```python
from build123d import *

# Parameters (mm, degrees)
SKETCH_1_W          = 35
SKETCH_1_H          = 10
SKETCH_1_R          = 2.1
EXTRUDE_1_DEPTH     = 2.5
EXTRUDE_2_DEPTH     = 2.5
SKETCH_2_3_R        = 1.6
CUT_EXTRUDE_1_DEPTH = 73.650942584
CHAMFER_1_SIZE      = 24.494897428
CHAMFER_1_SIZE_2    = 30
FILLET_1_R          = 2


with BuildPart() as part:
    # 草图1 → 凸台-拉伸1 (new body)
    with BuildSketch(Plane(origin=(0, 0, 0), x_dir=(1, 0, 0), z_dir=(0, 1, 0))):
        Rectangle(SKETCH_1_W, SKETCH_1_H)
        with Locations(Location((-7.5, 0, 0), (0, 0, 270))):
            Circle(SKETCH_1_R, mode=Mode.SUBTRACT)
        with Locations(Location((7.5, 0, 0), (0, 0, 270))):
            Circle(SKETCH_1_R, mode=Mode.SUBTRACT)
    extrude(amount=EXTRUDE_1_DEPTH)

    # 草图2 → 凸台-拉伸2 (add)
    with BuildSketch(Plane(origin=(0, 2.5, 0), x_dir=(1, 0, 0), z_dir=(0, 1, 0))):
        Polygon((-63.004240202, 2.548597579), (-52.651478398, -36.088435473), (17.5, -17.291403488), (17.5, -5), (-17.5, -5), (-17.5, 14.741421993), align=None)
    extrude(amount=-EXTRUDE_2_DEPTH)

    # 草图2<3> → 切除-拉伸1 (cut, through all)
    with BuildSketch(Plane(origin=(0, 2.5, 0), x_dir=(1, 0, 0), z_dir=(0, 1, 0))):
        with Locations(Location((-30.144179737, -4.175718463, 0), (0, 0, 270))):
            Circle(SKETCH_2_3_R)
        with Locations(Location((-24.967798835, -23.494234988, 0), (0, 0, 270))):
            Circle(SKETCH_2_3_R)
    extrude(amount=-CUT_EXTRUDE_1_DEPTH, mode=Mode.SUBTRACT)

    # 倒角1
    # the kernel refuses this chamfer: 30, 24.494897428 mm, written as the material it takes off along each edge
    with BuildSketch(Plane(origin=(-17.5, 79.650489639, -14.741421993), x_dir=(0.04137655931612181, 0, 0.999143623479207), z_dir=(0, -1, 0))) as chamfer_1_piece_1_section:
        Polygon((CHAMFER_1_SIZE * 0.999143623472, CHAMFER_1_SIZE * 0.0413765593158), (CHAMFER_1_SIZE_2 * 0.218630711303, CHAMFER_1_SIZE_2 * 0.975807671662), (0, 0), align=None)
    chamfer_1_piece_1 = extrude(amount=156.800979278, mode=Mode.PRIVATE)
    chamfer_1_piece_1 = split(chamfer_1_piece_1, bisect_by=Plane(origin=(-28.937603514, 1.25, -5), z_dir=(0, 0, -1)), keep=Keep.TOP, mode=Mode.PRIVATE)
    add(chamfer_1_piece_1, mode=Mode.SUBTRACT)

    # 圆角1
    fillet_1_edges = [part.edges().sort_by_distance(p)[0] for p in [
        (17.5, 1.25, 17.291403488),
        (-52.651478398, 1.25, 36.088435473),
        (-63.004240202, 1.25, -2.548597579),
        (-46.477774789, 1.25, -6.97685064),
        (-43.053769041, 1.25, -5),
        (17.5, 1.25, -5),
    ]]
    fillet(fillet_1_edges, radius=FILLET_1_R)


solid = part.part
```
Geometry: final body of the model. Coordinates: model frame, mm. A direction names the side the tool comes from. Give positions to 0.01 mm unless a question says otherwise; leave off trailing zeros. Order: outer loops, then holes, each group sorted by start corner. A loop starts at its lowest first (then second) coordinate and runs counter-clockwise, first axis right, second up. Notation, with made-up numbers: M 8.25,9 L 65.25,9 A10 ccw 65.25,23 Z; hole C 37,59.25 d3. An arc over 180 degrees is marked long. Answer as CSV lines item,"result". Start each with the question number.
1) Cut plane A-A (x = -31). Output: boundary loops of the cut face in (y, z).
2) Line query: line 1 (X direction, y = 0.4, z = -1.5); line 2 (Z direction, x = -24, y = 0.3); line 3 (X direction, y = 0.8, z = 16). Output: solid intervals per line, ascending. Write a range as from..to.
3) Cut plane C-C (x = 7.5). Output: boundary loops of the cut face in (y, z), then the cut area to 3 significant figures.
4) Cut plane D-D (z = 11.5). Output: boundary loops of the cut face in (x, y), then the cut area to 3 significant figures.
5) Set-up query: faces 1 (the cylindrical face through (-28.558, 1.268, 3.967)), 2 (the flat face through (-13, 1, -5)). Return all of +Z, -Z, +X, -X, +Y, -Y with unobstructed straight access to the full face (end or side cutting, diameter ignored); none if empty.
6) Cut plane B-B (y = 1.85). Output: boundary loops of the cut face in (x, z).
7) Mould query, pull axis X, two halves, no side actions, for faces 3 (the flat face through (-23, 2.5, 9)), 4 (the cylindrical face through (9.582, 1.232, -0.273)), 5 (the flat face through (17.5, 1, 7)). Classes: +X half, -X half, draft (parallel to the pull), parting line (faces both ways), or undercut.
8) First-contact query: P1, Ø1.2, axis at x = -7, y = 1.5, coming from the -Z side. Flat tip, straight axial feed; report the tip coordinate or a pass-through.
Findings below:
1,outline,"M 0,-5 L 2.5,-5 L 2.5,2.82 L 0,2.82 Z; M 0,5.53 L 2.5,5.53 L 2.5,30.29 L 0,30.29 Z"
2,line 1,"x = -62.52..-8.97, -6.03..6.03, 8.97..17.5"
2,line 2,"z = -5..22.22, 24.77..28.41"
2,line 3,"x = -58.03..17.49"
3,outline,"M 0,-5 L 2.5,-5 L 2.5,-2.1 L 0,-2.1 Z; M 0,2.1 L 2.5,2.1 L 2.5,19.97 L 0,19.97 Z"
3,area,"51.9 mm²"
4,outline,"M -59.24,0 L 17.5,0 L 17.5,2.5 L -59.24,2.5 Z"
4,area,"192 mm²"
5,face 1,"+Y, -Y"
5,face 2,"-Z, +X, +Y, -Y"
6,outline,"M -62.49,-0.62 A2 ccw -61.07,-3.07 L -47.28,-6.76 A2 ccw -45.76,-6.56 L -43.52,-5.27 A2 cw -42.52,-5 L 15.5,-5 A2 ccw 17.5,-3 L 17.5,15.76 A2 ccw 16.02,17.69 L -50.72,35.57 A2 ccw -53.17,34.16 Z; hole C -30.14,4.18 d3.2; hole C -24.97,23.49 d3.2; hole C -7.5,0 d4.2; hole C 7.5,0 d4.2"
7,face 3,"draft"
7,face 4,"undercut"
7,face 5,"+X half"
8,P1,"stops at z = -5"
